Autodesk Fusion 360 part; units mm, degrees
sketch "Sketch1" plane through (0, 0, 0) normal (0, 0, 1) x (1, 0, 0)
  line L0 (0, 0) -> (58.025, 0)
  line L1 (58.025, 0) -> (58.025, 79.025)
  line L2 (58.025, 79.025) -> (0, 79.025)
  line L3 (0, 79.025) -> (0, 0)
  line L4 (-9.5, -9.5) -> (67.525, -9.5)
  line L5 (67.525, -9.5) -> (67.525, 88.525)
  line L6 (67.525, 88.525) -> (-9.5, 88.525)
  line L7 (-9.5, 88.525) -> (-9.5, -9.5)
  circle A0 centre (-4.5, -4.5) radius 1.7
  circle A1 centre (-4.5, 83.525) radius 1.7
  circle A2 centre (62.525, 83.525) radius 1.7
  circle A3 centre (-4.5, -4.5) radius 3
  circle A4 centre (62.525, -4.5) radius 1.7
  circle A5 centre (62.525, -4.5) radius 3
  circle A6 centre (-4.5, 83.525) radius 3
  circle A7 centre (62.525, 83.525) radius 3
  dimension "d1" = 58.025
  dimension "d2" = 79.025
  dimension "d3" = 77.025
  dimension "d4" = 98.025
  dimension "d5" = 9.5
  dimension "d6" = 9.5
  dimension "d11" = 3.4
  dimension "d12" = 5
  dimension "d13" = 5
  dimension "d14" = 3.4
  dimension "d15" = 5
  dimension "d16" = 5
  dimension "d17" = 3.4
  dimension "d18" = 5
  dimension "d19" = 5
  dimension "d20" = 6
  dimension "d21" = 3.4
  dimension "d22" = 5
  dimension "d23" = 5
  dimension "d24" = 6
  dimension "d25" = 6
  dimension "d26" = 6
extrude "Extrude1" add sketch "Sketch1" along normal blind 9.9 from surface at 3.1 contours A3 | A5 | A6 | A7 makes body 1 at (59.7606, 82.3597, 9.7) makes body 2 at (-1.5037, -4.6495, 9.7) makes body 3 at (-7.0599, 81.9607, 9.7) makes body 4 at (65.5213, -4.6495, 9.7)
extrude "Extrude2" add sketch "Sketch1" along normal blind 13 contours L4 L5 L6 L7 bodies 1 2 3 4
extrude "Extrude3" add sketch "Sketch1" along normal blind 3 contours L0 L1 L2 L3 bodies 1
sketch "Sketch3" plane through (0, 0, 13) normal (0, 0, 1) x (-1, 0, 0)
  circle A0 centre (-62.525, -83.525) radius 1.7
  circle A1 centre (-62.525, 4.5) radius 1.7
  line L0 (0, 0) -> (0, -79.025)
  line L1 (0, -79.025) -> (-58.025, -79.025)
  line L2 (-58.025, -79.025) -> (-58.025, 0)
  line L3 (-58.025, 0) -> (0, 0)
  line L4 (9.5, -88.525) -> (9.5, 9.5)
  line L5 (9.5, 9.5) -> (-67.525, 9.5)
  line L6 (-67.525, 9.5) -> (-67.525, -88.525)
  line L7 (-67.525, -88.525) -> (9.5, -88.525)
  circle A2 centre (4.5, 4.5) radius 1.7
  circle A3 centre (4.5, -83.525) radius 1.7
  line L8 (-19.7, -88.525) -> (-38.2, -88.525)
  line L9 (-38.2, -88.525) -> (-38.2, -79.025)
  line L10 (-38.2, -79.025) -> (-19.7, -79.025)
  line L11 (-19.7, -79.025) -> (-19.7, -88.525)
  line L12 (9.5, -88.525) -> (9.5, 9.5)
  dimension "d36" = 18.5
  dimension "d37" = 29.2
extrude "Extrude4" cut sketch "Sketch3" against normal blind 7.5 contours L1 L7 L8 L9 L10 L11 bodies 1
fillet "Fillet1" radius 5 1 edges at (67.525, -9.5, 6.5) on bodies 1
fillet "Fillet2" radius 5 3 edges at (-9.5, -9.5, 6.5) (67.525, 88.525, 6.5) (-9.5, 88.525, 6.5) on bodies 1
Read the model definition and answer for the solid it produces. Units are mm, in the model's axes. A direction names the side the tool comes from. Coordinates: 2 decimals unless noted, no trailing zeros. Loops run counter-clockwise (first coordinate to the right, second up) from the corner with the lowest first, then second, coordinate; pieces in that order, holes last.
Q1. The part is cut by section B-B on x = 26.5. Write down the section's boundary in (y, z) (3 decimals).
Q2. Each of these flat-tipped pins is pushed along its axis until it touches: pin 1 Ø1 at (x, y) = (29.5, 27.5) entering from +Z; pin 2 Ø5 at (x, y) = (33, 85) entering from +Z; pin 3 Ø1.8 at (x, y) = (-3.5, 82.5) entering from -Z. Where does it stop, or does it pass through?
Q3. The mould has two halves that part along X. Classify faces 6 (the face through (66.021, -8.074, 6.591)), 7 (the face through (-8.07, -8, 6.59)), 8 (the face through (29, 84, 5.5)): +X half, -X half, draft (parallel to the pull), parting line (faces both ways), or undercut.
Q4. The part is cut by section C-C on y = 34. Write down the section's boundary in (x, z) (3 decimals).
Q5. Consider probe 1 along Y at (x, z) = (-4.5, 8.5) (3 decimals); probe 2 along Y at (x, z) = (57.5, 12.25) (3 decimals); probe 3 along X at (y, z) = (76, 10.5) (3 decimals). Determine where each line is inside the solid, lowest interval first.
Q6. Which of the six approach directions +Z, -Z, +X, -X, +Y, -Y give full straight-line access (tool end or side, diameter ignored) to faces 1 (the face through (29, 0, 8)), 2 (the face through (-3, 82, 3.1)), 3 (the face through (19.7, 84, 9)), 4 (the face through (66.1, 87.02, 6.59)), 5 (the face through (-7.996, 87.099, 6.591))?
Q7. The part is cut by section A-A on z = 7.25. Write down the section's boundary in (x, y) (3 decimals).
Results below:
1. outline: (-9.5, 0) - (88.525, 0) - (88.525, 5.5) - (79.025, 5.5) - (79.025, 3) - (0, 3) - (0, 13) - (-9.5, 13) - close
2. pin 1: stops at z = 3
2. pin 2: stops at z = 5.5
2. pin 3: stops at z = 3.1
3. face 6: +X half
3. face 7: -X half
3. face 8: undercut
4. outline: (-9.5, 0) - (67.525, 0) - (67.525, 13) - (58.025, 13) - (58.025, 3) - (0, 3) - (0, 13) - (-9.5, 13) - close
5. probe 1: y = -9.5 to -6.2, -2.8 to 81.825, 85.225 to 88.525
5. probe 2: y = -9.5 to 0, 79.025 to 88.525
5. probe 3: x = -9.5 to 0, 58.025 to 67.525
6. face 1: +Z
6. face 2: -Z
6. face 3: +Z, +Y
6. face 4: +Z, -Z, +X, +Y
6. face 5: +Z, -Z, -X, +Y
7. outline: (-9.5, -4.5) arc R5 ccw to (-4.5, -9.5) - (62.525, -9.5) arc R5 ccw to (67.525, -4.5) - (67.525, 83.525) arc R5 ccw to (62.525, 88.525) - (38.2, 88.525) - (38.2, 79.025) - (58.025, 79.025) - (58.025, 0) - (0, 0) - (0, 79.025) - (19.7, 79.025) - (19.7, 88.525) - (-4.5, 88.525) arc R5 ccw to (-9.5, 83.525) - close; hole circle Ø3.4 at (-4.5, -4.5); hole circle Ø3.4 at (-4.5, 83.525); hole circle Ø3.4 at (62.525, -4.5); hole circle Ø3.4 at (62.525, 83.525)
